Work out the finished part from the listing and answer in its coordinate system (mm). Face numbers are marked on the shaded views. Round coordinates to 2 decimals unless told otherwise and drop trailing zeros. Write each loop counter-clockwise with the first axis right and the second up, starting at its lowest first coordinate (ties: lowest second). Pieces come first, ordered by that corner, then holes. Notation, with made-up numbers: (-7.75, 4) - (0.25, 4) arc R15 cw to (0.25, 28) - close; hole circle Ø5 at (-32.75, -32.5). An arc over 180 degrees is marked (long way). Answer as a JSON object with one key per item and string values.
```python
from build123d import *

# Parameters (mm, degrees)
SKETCH_1_R               = 11.5
SKETCH_1_R_2             = 9.5
EXTRUDE_1_DEPTH          = 200
EXTRUDE_2_DEPTH          = 5
EXTRUDE_2_DEPTH_BACK     = 205
SKETCH_3_W               = 25
SKETCH_3_H               = 80
CUT_EXTRUDE_1_DEPTH      = 4
SKETCH_4_R               = 1
CUT_EXTRUDE_2_DEPTH      = 81
CUT_EXTRUDE_2_DEPTH_BACK = 4


with BuildPart() as part:
    # 草图1 → 凸台-拉伸1 (new body)
    with BuildSketch(Plane.XY):
        with BuildLine():
            ThreePointArc((0, -11.5), (-8.131727984, -8.131727984), (-11.5, 0))
            Line((-11.5, 0), (-11.5, -2.5))
            ThreePointArc((-11.5, -2.5), (-12.671572875, -5.328427125), (-15.5, -6.5))
            Line((-15.5, -6.5), (-99, -6.5))
            ThreePointArc((-99, -6.5), (-99.707106781, -6.792893219), (-100, -7.5))
            Line((-100, -7.5), (-100, -10.5))
            ThreePointArc((-100, -10.5), (-99.707106781, -11.207106781), (-99, -11.5))
            Line((-99, -11.5), (0, -11.5))
        make_face()
        Circle(SKETCH_1_R)
        Circle(SKETCH_1_R_2, mode=Mode.SUBTRACT)
    extrude(amount=EXTRUDE_1_DEPTH)

    # 草图2 → 凸台-拉伸2 (add, two sides)
    with BuildSketch(Plane(origin=(0, 0, 0), x_dir=(-1, 0, 0), z_dir=(0, 0, -1))) as extrude_2_sk:
        with BuildLine():
            Line((11.5, -2.5), (11.5, 0))
            ThreePointArc((11.5, 0), (8.131727984, -8.131727984), (0, -11.5))
            Line((0, -11.5), (99, -11.5))
            ThreePointArc((99, -11.5), (99.707106781, -11.207106781), (100, -10.5))
            Line((100, -10.5), (100, -7.5))
            ThreePointArc((100, -7.5), (99.707106781, -6.792893219), (99, -6.5))
            Line((99, -6.5), (15.5, -6.5))
            ThreePointArc((15.5, -6.5), (12.671572875, -5.328427125), (11.5, -2.5))
        make_face()
    extrude(amount=EXTRUDE_2_DEPTH)
    extrude(extrude_2_sk.sketch, amount=-EXTRUDE_2_DEPTH_BACK)

    # 草图3 → 切除-拉伸1 (cut)
    with BuildSketch(Plane(origin=(0, -6.5, 0), x_dir=(1, 0, 0), z_dir=(0, 1, 0))):
        with Locations((-57.5, -100)):
            Rectangle(SKETCH_3_W, SKETCH_3_H)
    extrude(amount=-CUT_EXTRUDE_1_DEPTH, mode=Mode.SUBTRACT)

    # 草图4 → 切除-拉伸2 (cut, two sides)
    with BuildSketch(Plane.XY.offset(60)) as cut_extrude_2_sk:
        with Locations((-68, -8.5)):
            Circle(SKETCH_4_R)
    extrude(amount=CUT_EXTRUDE_2_DEPTH, mode=Mode.SUBTRACT)
    extrude(cut_extrude_2_sk.sketch, amount=-CUT_EXTRUDE_2_DEPTH_BACK, mode=Mode.SUBTRACT)


solid = part.part
```
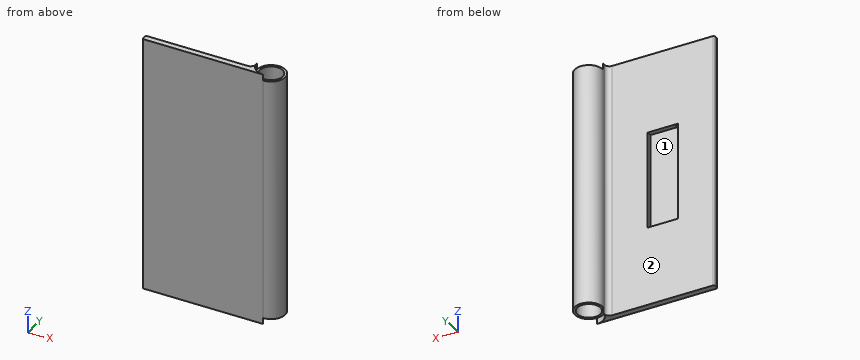
Item 1: Each of these flat-tipped pins is pushed along its axis until it touches: P1, Ø6, axis at y = -5.5, z = 45, coming from the +X side (3 decimals); P2, Ø4, axis at y = 5.5, z = 33, coming from the +X side; P3, Ø2, axis at y = -3, z = 142.5, coming from the -X side. Where does it stop, or does it pass through?
Results found:
{"P1": "x = 11.225", "P2": "x = 10.95", "P3": "x = -11.79"}
Item 2: A cutting plane is placed at A-A (z = 166.5). Write down the section's boundary in (x, y).
Results found:
{"outline": "(-100, -10.5) arc R1 ccw to (-99, -11.5) - (0, -11.5) arc R11.5 ccw (long way) to (-11.5, 0) - (-11.5, -2.5) arc R4 cw to (-15.5, -6.5) - (-99, -6.5) arc R1 ccw to (-100, -7.5) - close; hole circle Ø19 at (0, 0)"}
Item 3: A cutting plane is placed at C-C (y = 5.75). Write down the section's boundary in (x, z).
Results found:
{"outline": "(-9.96, 0) - (-7.56, 0) - (-7.56, 200) - (-9.96, 200) - close; (7.56, 0) - (9.96, 0) - (9.96, 200) - (7.56, 200) - close"}
Item 4: A cutting plane is placed at B-B (x = -48). Write down the section's boundary in (y, z), and give its area (3 significant figures).
Results found:
{"outline": "(-11.5, -5) - (-6.5, -5) - (-6.5, 60) - (-10.5, 60) - (-10.5, 140) - (-6.5, 140) - (-6.5, 205) - (-11.5, 205) - close", "area": "730 mm²"}
Item 5: Consider line 1 along Z through (x, y) = (-53, -7.5); line 2 along X through (y, z) = (-0.5, 160); line 3 along X through (y, z) = (-8.5, 140.55). Determine where each line is inside the solid, lowest interval first.
Results found:
{"line 1": "-5 to 60, 140 to 205", "line 2": "-11.5 to -9.49, 9.49 to 11.49", "line 3": "-100 to -69, -67 to -4.24, 4.24 to 7.75"}
Item 6: A cutting plane is placed at D-D (x = -3). Write down the section's boundary in (y, z), and give its area (3 significant figures).
Results found:
{"outline": "(-11.5, -5) - (-11.1, -5) - (-11.1, 0) - (-9.01, 0) - (-9.01, 200) - (-11.1, 200) - (-11.1, 205) - (-11.5, 205) - close; (9.01, 0) - (11.1, 0) - (11.1, 200) - (9.01, 200) - close", "area": "919 mm²"}
Item 7: Determine the mould class of the marked faces 1 and 2 for opening direction Z: pulls with the +Z half, pulls with the -Z half, needs draft (parallel to the pull), parting line crosses it, or undercut.
Results found:
{"face 1": "undercut", "face 2": "needs draft"}
